Design review of the part built by this model. Coordinates are the model's own, in mm. A direction names the side the tool comes from. Give positions to 0.01 mm unless a question says otherwise; leave off trailing zeros. Order: outer loops, then holes, each group sorted by start corner. A loop starts at its lowest first (then second) coordinate and runs counter-clockwise, first axis right, second up. Notation, with made-up numbers: M 87,1 L 139,1 A35 ccw 139,40 Z; hole C 88.25,6.5 d1. An arc over 180 degrees is marked long. Answer as a JSON object with one key per item and string values.
from build123d import *

# Parameters (mm, degrees)
SKETCH1_R                   = 74.5
SKETCH1_R_2                 = 72.5
EXTRUDE1_DEPTH              = 67.31
EXTRUDE2_START              = 24.511
SKETCH2_R                   = 127
SKETCH2_R_2                 = 72.5
EXTRUDE2_DEPTH              = 24.511
CUT_EXTRUDE1_REACH          = 203.715
SKETCH3_R                   = 4.2
CIRPATTERN1_COUNT           = 24
EXTRUDE3_START              = -2
SKETCH4_R                   = 74.5
SKETCH4_R_2                 = 32.2
EXTRUDE3_DEPTH              = 2
SKETCH13_R                  = 7.9375
EXTRUDE4_DEPTH              = 211.405273701
SKETCH14_R                  = 9.4996
SKETCH14_R_2                = 7.9375
EXTRUDE5_DEPTH              = 17.78
SKETCH15_R                  = 16.891
SKETCH15_R_2                = 7.9375
EXTRUDE6_DEPTH              = 7.239
SKETCH16_R                  = 2.1844
EXTRUDE7_DEPTH              = 7.239
CIRPATTERN2_COUNT           = 6
SKETCH17_W                  = 6.858832098
SKETCH17_H                  = 3.977015868
EXTRUDE8_DEPTH              = 7.62
MIRROR4_COPY_1_SKETCH_W     = 6.858832098
MIRROR4_COPY_1_SKETCH_H     = 3.977015868
MIRROR4_COPY_1_DEPTH        = 7.62
F_1_4_20_TAPPED_HOLE1_D     = 5.1054
F_1_4_20_TAPPED_HOLE1_DEPTH = 12.7
F_1_4_20_TAPPED_HOLE1_TIP   = 1.533816902
SKETCH21_W                  = 2.54
SKETCH21_H                  = 27.464757855
EXTRUDE9_DEPTH              = 1.27


with BuildPart() as part:
    # Sketch1 → Extrude1 (new body)
    with BuildSketch(Plane.XY):
        Circle(SKETCH1_R)
        Circle(SKETCH1_R_2, mode=Mode.SUBTRACT)
    extrude(amount=-EXTRUDE1_DEPTH)

    # Sketch2 → Extrude2 (add)
    with BuildSketch(Plane.XY.offset(EXTRUDE2_START)):
        Circle(SKETCH2_R)
        Circle(SKETCH2_R_2, mode=Mode.SUBTRACT)
    extrude(amount=-EXTRUDE2_DEPTH)

    # Sketch3 → Cut-Extrude1 (cut, up to next)
    with BuildSketch(Plane.XY.offset(24.511), mode=Mode.PRIVATE) as cut_extrude1_sk1:
        with Locations((15.131327149, -114.933840422)):
            Circle(SKETCH3_R)
    cut_extrude1_tool1 = extrude(cut_extrude1_sk1.sketch, amount=-CUT_EXTRUDE1_REACH, mode=Mode.PRIVATE) & part.part
    cut_extrude1 = cut_extrude1_tool1.solids().sort_by_distance((15.131327, -114.93384, 24.511))[0]
    add(cut_extrude1, mode=Mode.SUBTRACT)

    # CirPattern1: Cut-Extrude1 ×24 about axis
    cirpattern1_axis = Axis((0, 0, 0), (0, 0, 1))
    for i in range(1, CIRPATTERN1_COUNT):
        add(cut_extrude1.rotate(cirpattern1_axis, i * 360 / CIRPATTERN1_COUNT), mode=Mode.SUBTRACT)

    # Sketch4 → Extrude3 (add)
    with BuildSketch(Plane(origin=(0, 0, -67.31), x_dir=(-1, 0, 0), z_dir=(0, 0, -1)).offset(EXTRUDE3_START)):
        with Locations(Location((0, 0, 0), (0, 0, 180))):
            Circle(SKETCH4_R)
        Circle(SKETCH4_R_2, mode=Mode.SUBTRACT)
    extrude(amount=EXTRUDE3_DEPTH)

    # Sketch5 → Revolve1 (revolve)
    with BuildSketch(Plane(origin=(0, 0, 0), x_dir=(1, 0, 0), z_dir=(0, 1, 0)), mode=Mode.PRIVATE) as revolve1_sk:
        Polygon((-32.2, 67.31), (-32.2, 55.31), (-31, 55.31), (-31, 61.31), (-25, 67.31), align=None)
    revolve(revolve1_sk.sketch.rotate(Axis((0, 0, 0), (0, 0, -1)), 180), axis=Axis((0, 0, 0), (0, 0, -1)))

    # Sketch11 → Cut-Revolve1 (revolve, cut)
    with BuildSketch(Plane(origin=(0, 0, 0), x_dir=(1, 0, 0), z_dir=(0, 1, 0)), mode=Mode.PRIVATE) as cut_revolve1_sk:
        Polygon((-31.7, 67.31), (-31.7, 61.317106781), (-25.707106781, 67.31), align=None)
    revolve(cut_revolve1_sk.sketch.rotate(Axis((0, 0, 0), (0, 0, -1)), 180), axis=Axis((0, 0, 0), (0, 0, -1)), mode=Mode.SUBTRACT)

    # Sketch13 → Extrude4 (cut, through all)
    with BuildSketch(Plane.XY.offset(42.291)):
        with Locations((0, -89.535)):
            Circle(SKETCH13_R)
    extrude(amount=-EXTRUDE4_DEPTH, mode=Mode.SUBTRACT)

    # Sketch14 → Extrude5 (add)
    with BuildSketch(Plane.XY.offset(42.291)):
        with Locations((0, -89.535)):
            Circle(SKETCH14_R)
        with Locations((0, -89.535)):
            Circle(SKETCH14_R_2, mode=Mode.SUBTRACT)
    extrude(amount=-EXTRUDE5_DEPTH)

    # Sketch15 → Extrude6 (add)
    with BuildSketch(Plane.XY.offset(42.291)):
        with Locations((0, -89.535)):
            Circle(SKETCH15_R)
        with Locations((0, -89.535)):
            Circle(SKETCH15_R_2, mode=Mode.SUBTRACT)
    extrude(amount=-EXTRUDE6_DEPTH)

    # Sketch16 → Extrude7 (cut)
    with BuildSketch(Plane.XY.offset(42.291)):
        with Locations((0, -76.0476)):
            Circle(SKETCH16_R)
    extrude7 = extrude(amount=-EXTRUDE7_DEPTH, mode=Mode.SUBTRACT)

    # CirPattern2: Extrude7 ×6 about axis
    cirpattern2_axis = Axis((0, -89.535, 0), (0, 0, 1))
    for i in range(1, CIRPATTERN2_COUNT):
        add(extrude7.rotate(cirpattern2_axis, i * 360 / CIRPATTERN2_COUNT), mode=Mode.SUBTRACT)

    # Sketch17 → Extrude8 (add)
    with BuildSketch(Plane(origin=(0, 0, -67.31), x_dir=(-1, 0, 0), z_dir=(0, 0, -1))):
        with Locations((-58, -26)):
            Rectangle(SKETCH17_W, SKETCH17_H)
    extrude8 = extrude(amount=EXTRUDE8_DEPTH)

    # Mirror3: Extrude8 across plane
    add(extrude8.mirror(Plane.ZX))

    # Mirror4: Extrude8 across plane
    add(extrude8.mirror(Plane(origin=(0, 0, 0), x_dir=(0, 0, 1), z_dir=(1, 0, 0))))

    # Mirror4 copy 1 sketch → Mirror4 copy 1 (add)
    with BuildSketch(Plane(origin=(0, 0, -67.31), x_dir=(1, 0, 0), z_dir=(0, 0, -1))):
        with Locations((-58, -26)):
            Rectangle(MIRROR4_COPY_1_SKETCH_W, MIRROR4_COPY_1_SKETCH_H)
    extrude(amount=MIRROR4_COPY_1_DEPTH)

    # 1/4-20 Tapped Hole1
    with Locations(Plane(origin=(62.861792847, -62.861792847, 24.511), x_dir=(1, 0, 0), z_dir=(0, 0, 1))):
        with Locations((0, 0), (-125.723585694, 0), (-151.761792847, 62.861792847), (-125.723585694, 125.723585694), (0, 125.723585694), (26.038207153, 62.861792847)):
            Hole(F_1_4_20_TAPPED_HOLE1_D / 2, depth=F_1_4_20_TAPPED_HOLE1_DEPTH)
            with Locations((0, 0, -(F_1_4_20_TAPPED_HOLE1_DEPTH + F_1_4_20_TAPPED_HOLE1_TIP / 2))):  # 118° drill point
                Cone(0, F_1_4_20_TAPPED_HOLE1_D / 2, F_1_4_20_TAPPED_HOLE1_TIP, mode=Mode.SUBTRACT)

    # Sketch21 → Extrude9 (cut)
    with BuildSketch(Plane(origin=(0, 0, 0), x_dir=(-1, 0, 0), z_dir=(0, 0, -1))):
        with Locations((0, -119.254869633)):
            Rectangle(SKETCH21_W, SKETCH21_H)
        with Locations((0, 119.254869633)):
            Rectangle(SKETCH21_W, SKETCH21_H)
    extrude(amount=-EXTRUDE9_DEPTH, mode=Mode.SUBTRACT)


solid = part.part
(1) Draft analysis for pull direction Y (two halves, no side actions). For faces 1 (the cylindrical face through (-2.1, -98.8, 29.9)), 2 (the cylindrical face through (-14.58, 110.77, 12.43)), 3 (the cylindrical face through (93.908, 66.845, 12.427)), state which applies: +Y half, -Y half, draft (parallel to the pull), parting line (faces both ways), or undercut.
Checked values:
{"face 1": "parting line", "face 2": "undercut", "face 3": "undercut"}
(2) Insertion check: pin 1 (0.8 mm diameter, centred on x = 0.5, y = -115, fed in from -Z); pin 2 (12 mm diameter, centred on y = 14, z = 18, fed in from -X); pin 3 (7.5 mm diameter, centred on x = -57, z = -69.5, fed in from +Y). Each pin has a flat end and moves straight along its axis. Give the tip position at first contact, or say it passes through.
Checked values:
{"pin 1": "stops at z = 1.27", "pin 2": "stops at x = -126.75", "pin 3": "stops at y = 51.37"}
(3) To check wall thickness, follow L1, parallel to Y at x = -117, z = 22.5; L2, parallel to Z at x = -108.5, y = 50.5; L3, parallel to Y at x = -66, z = -9.5. State the ranges of each line that lie inside material, in increasing order. Write a range as from..to.
Checked values:
{"L1": "y = -49.4..-18.79, -11.47..11.47, 18.79..49.4", "L2": "z = 0..24.51", "L3": "y = -34.56..-30, 30..34.56"}
(4) Tool access review of faces 4 (the cylindrical face through (-68.01, -88.64, 12.43)), 5 (the flat face through (-58, 24.011, -71)), 6 (the cylindrical face through (-4.036, -30.736, -58.352)): name each direction out of +Z, -Z, +X, -X, +Y, -Y from which nothing blocks a thin tool from reaching the whole face with its end or side.
Checked values:
{"face 4": "+Z, -Z", "face 5": "-Z, +X, -X", "face 6": "+Z"}
(5) We need section A-A (z = -36.5). Write out the cut boundary in (x, y), plus the area to 3 significant figures.
Checked values:
{"outline": "C 0,0 d149; hole C 0,0 d145", "area": "924 mm^2"}
